```python
from build123d import *

# Parameters (mm, degrees)
SKETCH_1_W             = 25
SKETCH_1_H             = 10
EXTRUDE_1_DEPTH        = 4
SKETCH_2_R             = 1.5
CUT_EXTRUDE_1_DEPTH    = 15.044571905
CUT_EXTRUDE_2_DEPTH    = 3
SKETCH_4_W             = 25
SKETCH_4_H             = 12.1
EXTRUDE_2_DEPTH        = 4
SKETCH_5_R             = 1.5
CUT_EXTRUDE_3_DEPTH    = 22.55597365
CUT_EXTRUDE_4_DEPTH    = 3
PATTERN_LINEAR_1_COUNT = 6
PATTERN_LINEAR_1_PITCH = 12.1
FILLET_1_R             = 5
FILLET_2_R             = 1


with BuildPart() as part:
    # 草图1 → 凸台-拉伸1 (new body)
    with BuildSketch(Plane.XY):
        Rectangle(SKETCH_1_W, SKETCH_1_H)
    extrude(amount=EXTRUDE_1_DEPTH)

    # 草图2 → 切除-拉伸1 (cut, through all)
    with BuildSketch(Plane.XY.offset(4)):
        Circle(SKETCH_2_R)
        with Locations((-8, 0)):
            Circle(SKETCH_2_R)
        with Locations(Location((8, 0, 0), (0, 0, 180))):
            Circle(SKETCH_2_R)
    extrude(amount=-CUT_EXTRUDE_1_DEPTH, mode=Mode.SUBTRACT)

    # 草图3 → 切除-拉伸2 (cut)
    with BuildSketch(Plane.XY.offset(4)):
        Polygon((-8, 3.175426481), (-10.75, 1.58771324), (-10.75, -1.58771324), (-8, -3.175426481), (-5.25, -1.58771324), (-5.25, 1.58771324), align=None)
        Polygon((0, 3.175426481), (-2.75, 1.58771324), (-2.75, -1.58771324), (0, -3.175426481), (2.75, -1.58771324), (2.75, 1.58771324), align=None)
        Polygon((8, 3.175426481), (5.25, 1.58771324), (5.25, -1.58771324), (8, -3.175426481), (10.75, -1.58771324), (10.75, 1.58771324), align=None)
    extrude(amount=-CUT_EXTRUDE_2_DEPTH, mode=Mode.SUBTRACT)

    # 草图4 → 凸台-拉伸2 (add)
    with BuildSketch(Plane.XY.offset(4)):
        with Locations((0, -11.05)):
            Rectangle(SKETCH_4_W, SKETCH_4_H)
    extrude_2 = extrude(amount=-EXTRUDE_2_DEPTH)

    # 草图5 → 切除-拉伸3 (cut, through all)
    with BuildSketch(Plane.XY.offset(4)):
        with Locations((0, -12.1)):
            Circle(SKETCH_5_R)
        with Locations((-8, -12.1)):
            Circle(SKETCH_5_R)
        with Locations(Location((8, -12.1, 0), (0, 0, 180))):
            Circle(SKETCH_5_R)
    cut_extrude_3 = extrude(amount=-CUT_EXTRUDE_3_DEPTH, mode=Mode.SUBTRACT)

    # 草图6 → 切除-拉伸4 (cut)
    with BuildSketch(Plane.XY.offset(4)):
        Polygon((-8, -8.924573519), (-10.75, -10.51228676), (-10.75, -13.68771324), (-8, -15.275426481), (-5.25, -13.68771324), (-5.25, -10.51228676), align=None)
        Polygon((0, -8.924573519), (-2.75, -10.51228676), (-2.75, -13.68771324), (0, -15.275426481), (2.75, -13.68771324), (2.75, -10.51228676), align=None)
        Polygon((8, -8.924573519), (5.25, -10.51228676), (5.25, -13.68771324), (8, -15.275426481), (10.75, -13.68771324), (10.75, -10.51228676), align=None)
    cut_extrude_4 = extrude(amount=-CUT_EXTRUDE_4_DEPTH, mode=Mode.SUBTRACT)

    # 阵列(线性)1: 凸台-拉伸2, 切除-拉伸3, 切除-拉伸4 ×6
    with Locations(*[(0, -i * PATTERN_LINEAR_1_PITCH, 0) for i in range(1, PATTERN_LINEAR_1_COUNT)]):
        add(extrude_2)
        add(cut_extrude_3, mode=Mode.SUBTRACT)
        add(cut_extrude_4, mode=Mode.SUBTRACT)

    # 圆角1
    fillet_1_edges = [part.edges().sort_by_distance(p)[0] for p in [
        (-12.5, -77.6, 2),
        (12.5, -77.6, 2),
        (-12.5, 5, 2),
        (12.5, 5, 2),
    ]]
    fillet(fillet_1_edges, radius=FILLET_1_R)

    # 圆角2
    fillet_2_edges = [part.edges().sort_by_distance(p)[0] for p in [
        (0, -77.6, 0),
        (0, -77.6, 4),
        (12.5, -36.3, 4),
        (0, 5, 4),
        (-12.5, -36.3, 4),
        (-11.035533906, -76.135533906, 4),
        (-11.035533906, 3.535533906, 4),
        (11.035533906, 3.535533906, 4),
        (11.035533906, -76.135533906, 4),
        (12.5, -36.3, 0),
        (-12.5, -36.3, 0),
        (0, 5, 0),
        (-11.035533906, -76.135533906, 0),
        (-11.035533906, 3.535533906, 0),
        (11.035533906, 3.535533906, 0),
        (11.035533906, -76.135533906, 0),
    ]]
    fillet(fillet_2_edges, radius=FILLET_2_R)


solid = part.part
```
The listing builds one solid part. Answer for the finished solid, in the listing's coordinates (mm). A direction names the side the tool comes from. Give positions to 0.01 mm unless a question says otherwise; leave off trailing zeros. Write each question's results on one line, items separated by ' | '.
Q1. For a pull along X with two mould halves and no side action, classify faces 1 (the flat face through (5.25, -36, 3)), 2 (the flat face through (-12.5, -37, 2)) as released by +X, released by -X, zero draft, split by the parting line, or undercut.
Output values:
face 1: undercut | face 2: released by -X
Q2. Flat-ended cylindrical pins translate along their axes: P1, Ø3, axis at x = 9.5, y = -49.5, coming from the -Z side; P2, Ø1.8, axis at x = 0, y = -60.5, coming from the +Z side; P3, Ø1.6, axis at x = -7, y = -49, coming from the +Z side. Find the tip coordinate at first contact, or state that the pin passes through.
Output values:
P1: z = 0 | P2: through | P3: z = 1
Q3. A tool of negligible diameter and unlimited length cuts with its end or side. For faces 3 (the flat face through (1.394, -21.83, 2.521)), 4 (the cylindrical face through (-9.5, 0.07, 0.51)), from which of +Z, -Z, +X, -X, +Y, -Y can it reach the whole face along a straight path? Write none if from no direction.
Output values:
face 3: +Z | face 4: +Z, -Z
Q4. Consider L1, parallel to X at y = -2, z = 2.75; L2, parallel to X at y = -72.6, z = 0.4; L3, parallel to Z at x = -10.25, y = -35. Determine where each line is inside the solid, lowest interval first. Write a range as from..to.
Output values:
L1: -12.5..-10.04, -5.96..-2.04, 2.04..5.96, 10.04..12.5 | L2: -12.3..-9.5, -6.5..-1.5, 1.5..6.5, 9.5..12.3 | L3: 0..1
Q5. Section A-A, the plane y = -12.1 is taken. Count the separate pieces of the cut face and the enclosed holes in it, then the cut area to 3 significant figures.
Output values:
separate pieces: 4 | enclosed holes: 0 | area: 40.6 mm2
